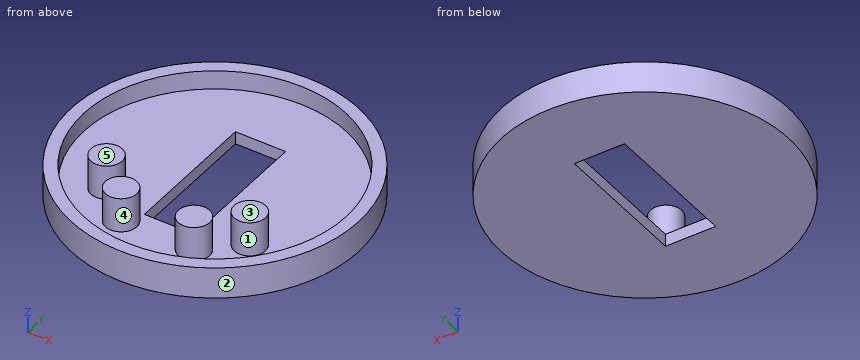
from build123d import *

# Parameters (mm, degrees)
SKIZZE2_W                       = 8
SKIZZE2_H                       = 22
SCHNITT_LINEAR_AUSTRAGEN1_DEPTH = 10
SKIZZE3_R                       = 2.5
AUFSATZ_LINEAR_AUSTRAGEN1_DEPTH = 7.5
SKIZZE3_5_R                     = 2.5
AUFSATZ_LINEAR_AUSTRAGEN2_DEPTH = 7.5
SKIZZE3_6_R                     = 2.5
AUFSATZ_LINEAR_AUSTRAGEN3_DEPTH = 7.5
SKIZZE3_7_R                     = 2.5
AUFSATZ_LINEAR_AUSTRAGEN4_DEPTH = 7.5


with BuildPart() as part:
    # Skizze1 → Rotation2 (revolve)
    with BuildSketch(Plane(origin=(0, 0, 0), x_dir=(1, 0, 0), z_dir=(0, 1, 0))):
        Polygon((0, 0), (22.902, 0), (22.902, -5), (20.902, -5), (20.902, -2), (0, -2), align=None)
    revolve(axis=Axis((0, 0, 2), (0, 0, -1)))

    # Skizze2 → Schnitt-Linear austragen1 (cut)
    with BuildSketch(Plane(origin=(0, 0, 0), x_dir=(-1, 0, 0), z_dir=(0, 0, -1))):
        Rectangle(SKIZZE2_W, SKIZZE2_H)
    extrude(amount=-SCHNITT_LINEAR_AUSTRAGEN1_DEPTH, mode=Mode.SUBTRACT)

    # Skizze3 → Aufsatz-Linear austragen1 (add)
    with BuildSketch(Plane.XY):
        with Locations((11.4275, -8.885)):
            Circle(SKIZZE3_R)
    extrude(amount=AUFSATZ_LINEAR_AUSTRAGEN1_DEPTH)

    # Skizze3_5 → Aufsatz-Linear austragen2 (add)
    with BuildSketch(Plane.XY):
        with Locations((5.8065, -13.863)):
            Circle(SKIZZE3_5_R)
    extrude(amount=AUFSATZ_LINEAR_AUSTRAGEN2_DEPTH)

    # Skizze3_6 → Aufsatz-Linear austragen3 (add)
    with BuildSketch(Plane.XY):
        with Locations((-5.8065, -13.863)):
            Circle(SKIZZE3_6_R)
    extrude(amount=AUFSATZ_LINEAR_AUSTRAGEN3_DEPTH)

    # Skizze3_7 → Aufsatz-Linear austragen4 (add)
    with BuildSketch(Plane.XY):
        with Locations((-11.4275, -8.885)):
            Circle(SKIZZE3_7_R)
    extrude(amount=AUFSATZ_LINEAR_AUSTRAGEN4_DEPTH)


solid = part.part
Part model, mm, in its own coordinate system. Face numbers are marked on the shaded views. A direction names the side the tool comes from. Coordinates: 2 decimals unless noted, no trailing zeros. Write each loop counter-clockwise with the first axis right and the second up, starting at its lowest first coordinate (ties: lowest second). Pieces come first, ordered by that corner, then holes. Notation, with made-up numbers: (76, 26) - (121, 26) arc R22 ccw to (121, 65) - close; hole circle Ø2 at (69.5, 65). An arc over 180 degrees is marked (long way). Put each result on its own line as item: value.
1. Band-saw the part on B-B (x = 0). Write the cut outline in (y, z), then the cut area to 3 significant figures.
Final values:
outline: (-22.9, 0) - (-11, 0) - (-11, 2) - (-20.9, 2) - (-20.9, 5) - (-22.9, 5) - close; (11, 0) - (22.9, 0) - (22.9, 5) - (20.9, 5) - (20.9, 2) - (11, 2) - close
area: 59.6 mm²
2. Two-plate mould, pull along Y, no slides. Class the marked faces 1, 2 and 3: +Y half, -Y half, draft (parallel to the pull), parting line (faces both ways), or undercut.
Final values:
face 1: undercut
face 2: parting line
face 3: draft
3. Flat gauge pins, fed straight in: pin 1 Ø3 at (x, y) = (17, -16.5) entering from +Z; pin 2 Ø1 at (y, z) = (5.5, 4) entering from -X; pin 3 Ø4 at (y, z) = (-17.5, 5) entering from +X. Where does each tip first touch, or does it go through?
Final values:
pin 1: stops at z = 5
pin 2: stops at x = -22.35
pin 3: stops at x = 16.86
4. 3-axis set-ups, long thin cutter, end or side, ignore diameter. For the marked faces 4 and 5: which of +Z, -Z, +X, -X, +Y, -Y reach the whole face in a straight line?
Final values:
face 4: +Z
face 5: +Z, +X, -X, +Y, -Y
5. Band-saw the part on A-A (y = 0). Write the cut outline in (x, z).
Final values:
outline: (-22.9, 0) - (-4, 0) - (-4, 2) - (-20.9, 2) - (-20.9, 5) - (-22.9, 5) - close; (4, 0) - (22.9, 0) - (22.9, 5) - (20.9, 5) - (20.9, 2) - (4, 2) - close
6. Band-saw the part on C-C (z = 4.25). Write the cut outline in (x, y) (1 decimal).
Final values:
outline: circle Ø45.8 at (0, 0); circle Ø5 at (-11.4, -8.9); circle Ø5 at (-5.8, -13.9); circle Ø5 at (5.8, -13.9); circle Ø5 at (11.4, -8.9); hole circle Ø41.8 at (0, 0)
7. Probe line 1 along Y through (x, z) = (0, 3.35); line 2 along X through (y, z) = (-7.5, 3.25). List the from-to ranges inside material, lowest first. Write a range as [from, to].
Final values:
line 1: y = [-22.9, -20.9], [20.9, 22.9]
line 2: x = [-21.64, -19.51], [-13.51, -9.35], [9.35, 13.51], [19.51, 21.64]
8. Band-saw the part on D-D (y = 15.5). Write the cut outline in (x, z), then the cut area to 3 significant figures.
Final values:
outline: (-16.86, 0) - (16.86, 0) - (16.86, 5) - (14.02, 5) - (14.02, 2) - (-14.02, 2) - (-14.02, 5) - (-16.86, 5) - close
area: 84.5 mm²
